```python
from build123d import *

# Parameters (mm, degrees)
SKETCH142_R               = 2.5
EXTRUDE046_DEPTH          = 19
EXTRUDE047_DEPTH          = 19
CYLINDER185_R             = 2
CYLINDER185_DEPTH         = 10
CYLINDER186_R             = 2
CYLINDER186_DEPTH         = 10
CYLINDER187_R             = 2
CYLINDER187_DEPTH         = 10
CYLINDER184_R             = 2
CYLINDER184_DEPTH         = 10
FUSION121_PLACEMENT_ANGLE = 45
CYLINDER180_R             = 2
CYLINDER180_DEPTH         = 10
CYLINDER181_R             = 2
CYLINDER181_DEPTH         = 10
CYLINDER182_R             = 2
CYLINDER182_DEPTH         = 10
CYLINDER183_R             = 2
CYLINDER183_DEPTH         = 10
CYLINDER170_R             = 2
CYLINDER170_DEPTH         = 10
CYLINDER171_R             = 2
CYLINDER171_DEPTH         = 10
CYLINDER172_R             = 2
CYLINDER172_DEPTH         = 10
CYLINDER169_R             = 2
CYLINDER169_DEPTH         = 10
FUSION111_PLACEMENT_ANGLE = 45
CYLINDER176_R             = 5
CYLINDER176_DEPTH         = 5.82
CYLINDER177_R             = 5
CYLINDER177_DEPTH         = 5.82
CYLINDER178_R             = 5
CYLINDER178_DEPTH         = 5.82
CYLINDER179_R             = 5
CYLINDER179_DEPTH         = 5.82
CYLINDER173_R             = 40
CYLINDER173_DEPTH         = 4.5
CYLINDER174_R             = 24
CYLINDER174_DEPTH         = 7
EXTRUDE044_DEPTH          = 33
SKETCH141_W               = 27
SKETCH141_H               = 14.5
SKETCH141_R               = 2.125
EXTRUDE045_DEPTH          = 4


with BuildPart() as lightwire:
    # Sketch142 → Extrude046 (new body)
    with BuildSketch(Plane.XY.offset(-24.25)):
        with Locations((18.5, -375)):
            Circle(SKETCH142_R)
    extrude(amount=EXTRUDE046_DEPTH)


with BuildPart() as extrude047:
    # Sketch143 → Extrude047 (new body)
    with BuildSketch(Plane.XY.offset(-24.25)):
        with BuildLine():
            ThreePointArc((18.5, -380), (23.5, -375), (18.5, -370))
            Line((13.5, -370), (18.5, -370))
            Line((13.5, -380), (13.5, -370))
            Line((18.5, -380), (13.5, -380))
        make_face()
    extrude(amount=EXTRUDE047_DEPTH)


with BuildPart() as obj1:
    # Cylinder185 → Cylinder185 (new body)
    with BuildSketch(Plane(origin=(35, 0, 65), x_dir=(1, 0, 0), z_dir=(0, 0, 1))):
        Circle(CYLINDER185_R)
    extrude(amount=CYLINDER185_DEPTH)


with BuildPart() as obj2:
    # Cylinder186 → Cylinder186 (new body)
    with BuildSketch(Plane(origin=(0, 35, 65), x_dir=(1, 0, 0), z_dir=(0, 0, 1))):
        Circle(CYLINDER186_R)
    extrude(amount=CYLINDER186_DEPTH)


with BuildPart() as obj3:
    # Cylinder187 → Cylinder187 (new body)
    with BuildSketch(Plane(origin=(0, -35, 65), x_dir=(1, 0, 0), z_dir=(0, 0, 1))):
        Circle(CYLINDER187_R)
    extrude(amount=CYLINDER187_DEPTH)


with BuildPart() as fusion121:
    # Cylinder184 → Cylinder184 (new body)
    with BuildSketch(Plane(origin=(-35, 0, 65), x_dir=(1, 0, 0), z_dir=(0, 0, 1))):
        Circle(CYLINDER184_R)
    extrude(amount=CYLINDER184_DEPTH)

    # Fusion121: union obj1, obj2, obj3
    add(obj1.part)
    add(obj2.part)
    add(obj3.part)


with BuildPart() as fusion121_1:
    # Fusion121 placement: moved
    add(fusion121.part.moved(Location((0, -374, -75))).rotate(Axis((0, -374, -75), (0, 0, -1)), FUSION121_PLACEMENT_ANGLE))


with BuildPart() as cylinder180:
    # Cylinder180 → Cylinder180 (new body)
    with BuildSketch(Plane(origin=(0, -21, 0), x_dir=(1, 0, 0), z_dir=(0, 0, 1))):
        Circle(CYLINDER180_R)
    extrude(amount=CYLINDER180_DEPTH)


with BuildPart() as m3heatsetcuts031:
    # Cylinder181 → Cylinder181 (new body)
    with BuildSketch(Plane(origin=(20.5, -21, 0), x_dir=(1, 0, 0), z_dir=(0, 0, 1))):
        Circle(CYLINDER181_R)
    extrude(amount=CYLINDER181_DEPTH)

    # Fusion118: union Cylinder180
    add(cylinder180.part)


with BuildPart() as m3heatsetcuts031_1:
    # Fusion118 placement: moved
    add(m3heatsetcuts031.part.moved(Location((-5, 39, 70))))


with BuildPart() as cylinder182:
    # Cylinder182 → Cylinder182 (new body)
    with BuildSketch(Plane(origin=(0, -21, 0), x_dir=(1, 0, 0), z_dir=(0, 0, 1))):
        Circle(CYLINDER182_R)
    extrude(amount=CYLINDER182_DEPTH)


with BuildPart() as m3heatsetcuts030:
    # Cylinder183 → Cylinder183 (new body)
    with BuildSketch(Plane(origin=(20.5, -21, 0), x_dir=(1, 0, 0), z_dir=(0, 0, 1))):
        Circle(CYLINDER183_R)
    extrude(amount=CYLINDER183_DEPTH)

    # Fusion119: union Cylinder182
    add(cylinder182.part)


with BuildPart() as m3heatsetcuts030_1:
    # Fusion119 placement: moved
    add(m3heatsetcuts030.part.moved(Location((-5, 3, 70))))

    # Fusion117: union m3HeatSetCuts031
    add(m3heatsetcuts031_1.part)


with BuildPart() as m3heatsetcuts030_2:
    # Fusion117 placement: moved
    add(m3heatsetcuts030_1.part.moved(Location((128.75, 10, -1))))


with BuildPart() as obj4:
    # Cylinder170 → Cylinder170 (new body)
    with BuildSketch(Plane(origin=(35, 0, 65), x_dir=(1, 0, 0), z_dir=(0, 0, 1))):
        Circle(CYLINDER170_R)
    extrude(amount=CYLINDER170_DEPTH)


with BuildPart() as obj5:
    # Cylinder171 → Cylinder171 (new body)
    with BuildSketch(Plane(origin=(0, 35, 65), x_dir=(1, 0, 0), z_dir=(0, 0, 1))):
        Circle(CYLINDER171_R)
    extrude(amount=CYLINDER171_DEPTH)


with BuildPart() as obj6:
    # Cylinder172 → Cylinder172 (new body)
    with BuildSketch(Plane(origin=(0, -35, 65), x_dir=(1, 0, 0), z_dir=(0, 0, 1))):
        Circle(CYLINDER172_R)
    extrude(amount=CYLINDER172_DEPTH)


with BuildPart() as fusion120:
    # Cylinder169 → Cylinder169 (new body)
    with BuildSketch(Plane(origin=(-35, 0, 65), x_dir=(1, 0, 0), z_dir=(0, 0, 1))):
        Circle(CYLINDER169_R)
    extrude(amount=CYLINDER169_DEPTH)

    # Fusion111: union obj4, obj5, obj6
    add(obj4.part)
    add(obj5.part)
    add(obj6.part)


with BuildPart() as fusion120_1:
    # Fusion111 placement: moved
    add(fusion120.part.moved(Location((0, -374, -75))).rotate(Axis((0, -374, -75), (0, 0, -1)), FUSION111_PLACEMENT_ANGLE))

    # Fusion120: union m3HeatSetCuts030
    add(m3heatsetcuts030_2.part)


with BuildPart() as cylinder176:
    # Cylinder176 → Cylinder176 (new body)
    with BuildSketch(Plane(origin=(0, -21, 0), x_dir=(1, 0, 0), z_dir=(0, 0, 1))):
        Circle(CYLINDER176_R)
    extrude(amount=CYLINDER176_DEPTH)


with BuildPart() as m3heatsetcuts027:
    # Cylinder177 → Cylinder177 (new body)
    with BuildSketch(Plane(origin=(20.5, -21, 0), x_dir=(1, 0, 0), z_dir=(0, 0, 1))):
        Circle(CYLINDER177_R)
    extrude(amount=CYLINDER177_DEPTH)

    # Fusion112: union Cylinder176
    add(cylinder176.part)


with BuildPart() as m3heatsetcuts027_1:
    # Fusion112 placement: moved
    add(m3heatsetcuts027.part.moved(Location((-5, 39, 70))))


with BuildPart() as cylinder178:
    # Cylinder178 → Cylinder178 (new body)
    with BuildSketch(Plane(origin=(0, -21, 0), x_dir=(1, 0, 0), z_dir=(0, 0, 1))):
        Circle(CYLINDER178_R)
    extrude(amount=CYLINDER178_DEPTH)


with BuildPart() as m3heatsetcuts029:
    # Cylinder179 → Cylinder179 (new body)
    with BuildSketch(Plane(origin=(20.5, -21, 0), x_dir=(1, 0, 0), z_dir=(0, 0, 1))):
        Circle(CYLINDER179_R)
    extrude(amount=CYLINDER179_DEPTH)

    # Fusion113: union Cylinder178
    add(cylinder178.part)


with BuildPart() as m3heatsetcuts029_1:
    # Fusion113 placement: moved
    add(m3heatsetcuts029.part.moved(Location((-5, 3, 70))))

    # Fusion114: union m3HeatSetCuts027
    add(m3heatsetcuts027_1.part)


with BuildPart() as m3heatsetcuts029_2:
    # Fusion114 placement: moved
    add(m3heatsetcuts029_1.part.moved(Location((128.75, 10, -1))))


with BuildPart() as base015:
    # Cylinder173 → Cylinder173 (new body)
    with BuildSketch(Plane(origin=(136, 0, 65), x_dir=(1, 0, 0), z_dir=(0, 0, 1))):
        Circle(CYLINDER173_R)
    extrude(amount=CYLINDER173_DEPTH)


with BuildPart() as basecut004:
    # Cylinder174 → Cylinder174 (new body)
    with BuildSketch(Plane(origin=(5, 0, 74), x_dir=(1, 0, 0), z_dir=(0, 0, 1))):
        Circle(CYLINDER174_R)
    extrude(amount=CYLINDER174_DEPTH)


with BuildPart() as lightmodule:
    # Sphere006 → Sphere006 (revolve)
    with BuildSketch(Plane(origin=(5, 0, 74), x_dir=(1, 0, 0), z_dir=(0, -1, 0))):
        with BuildLine():
            ThreePointArc((27.5, 0), (27.349352, 2.874533), (26.899059, 5.717571))
            Line((26.899059, 5.717571), (0, 5.717571))
            Line((0, 5.717571), (0, 0))
            Line((0, 0), (27.5, 0))
        make_face()
    revolve(axis=Axis((5, 0, 74), (0, 0, 1)))

    # Cut058: cut baseCut004
    add(basecut004.part, mode=Mode.SUBTRACT)


with BuildPart() as lightmodule_1:
    # Cut058 placement: moved
    add(lightmodule.part.moved(Location((131, 0, -5))))

    # Fusion115: union base015
    add(base015.part)


with BuildPart() as lightmodule_2:
    # Fusion115 placement: moved
    add(lightmodule_1.part.moved(Location((-2, 10, 0))))

    # Fusion116: union m3HeatSetCuts029
    add(m3heatsetcuts029_2.part)

    # Cut059: cut Fusion120
    add(fusion120_1.part, mode=Mode.SUBTRACT)


with BuildPart() as lightmodule_3:
    # Cut059 placement: moved
    add(lightmodule_2.part.moved(Location((-134, -384, -74.75))))

    # Cut060: cut Fusion121
    add(fusion121_1.part, mode=Mode.SUBTRACT)


with BuildPart() as extrude044:
    # Sketch140 → Extrude044 (new body)
    with BuildSketch(Plane.XZ.offset(370)):
        Polygon((-13.5, -9.75), (-9.5, -9.75), (-9.5, -20.25), (9.5, -20.25), (9.5, -9.75), (13.5, -9.75), (13.5, -24.25), (-13.5, -24.25), align=None)
    extrude(amount=EXTRUDE044_DEPTH)


with BuildPart() as lightmodule015:
    # Sketch141 → Extrude045 (new body)
    with BuildSketch(Plane.XZ.offset(403)):
        with Locations((0, -17)):
            Rectangle(SKETCH141_W, SKETCH141_H)
        with Locations((0, -15)):
            Circle(SKETCH141_R, mode=Mode.SUBTRACT)
    extrude(amount=EXTRUDE045_DEPTH)

    # Fusion122: union lightModule, Extrude044
    add(lightmodule_3.part)
    add(extrude044.part)

    # Fusion123: union Extrude047
    add(extrude047.part)

    # Cut061: cut lightWire
    add(lightwire.part, mode=Mode.SUBTRACT)


solid = lightmodule015.part
```
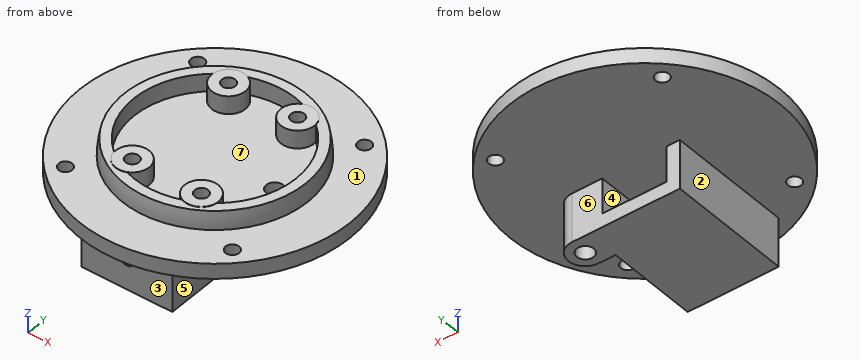
The model under review builds one solid part; all positions refer to its coordinate system, in mm. Face numbers are marked on the shaded views. A direction names the side the tool comes from. Give positions to 0.01 mm unless a question says otherwise; leave off trailing zeros. Write each loop counter-clockwise with the first axis right and the second up, starting at its lowest first coordinate (ties: lowest second). Pieces come first, ordered by that corner, then holes. Notation, with made-up numbers: (65, -13.5) -> (117, -13.5) arc R11 ccw to (117, 1.5) -> close; hole circle Ø5 at (74, 29). An arc over 180 degrees is marked (long way). Put each result on its own line as item: value.
(1) For pin 1 Ø4.5 at (x, y) = (-24.75, -349.25) entering from -Z; pin 2 Ø3 at (x, z) = (4, -4.5) entering from +Y; pin 3 Ø2 at (x, y) = (-28, -387.5) entering from +Z, all flat-tipped, find the tip position at first contact; note any pin that passes through.
Results are:
pin 1: z = -9.75
pin 2: y = -334.09
pin 3: z = -5.25
(2) We need section C-C, the plane y = -342. Give the boundary of the cut face in (x, z), and give its area (3 significant figures).
Results are:
outline: (-24, -9.75) -> (24, -9.75) -> (24, -5.25) -> (-24, -5.25) -> close
area: 216 mm²
(3) We need section B-B, the plane y = -375. State how many separate pieces and enclosed holes the cut face has, and give its area (3 significant figures).
Results are:
separate pieces: 2
enclosed holes: 1
area: 636 mm²
(4) The part is to be moulded in two halves that separate along X. For the marked faces 5, 6 and 7, say which applies: pulls with the +X half, pulls with the -X half, needs draft (parallel to the pull), parting line crosses it, or undercut.
Results are:
face 5: pulls with the +X half
face 6: needs draft
face 7: undercut
(5) We need section D-D, the plane x = 29.5. Give the boundary of the cut face in (y, z).
Results are:
outline: (-401.01, -9.75) -> (-346.99, -9.75) -> (-346.99, -5.25) -> (-401.01, -5.25) -> close
(6) To check wall thickness, follow probe 1 along Z at (x, y) = (-6, -388); probe 2 along Y at (x, z) = (-23.5, -7); probe 3 along Y at (x, z) = (18.5, -16). State the ranges of each line that lie inside material, in increasing order. Write a range as from..to.
Results are:
probe 1: -24.25..-20.25, -9.75..-5.25
probe 2: -406.37..-400.31, -397.19..-350.81, -347.69..-341.63
probe 3: -380..-377.5, -372.5..-370
(7) Tool access review of the marked faces 1, 2, 3 and 4: name each direction out of +Z, -Z, +X, -X, +Y, -Y from which nothing blocks a thin tool from reaching the whole face with its end or side.
Results are:
face 1: +Z
face 2: -Z, -X, +Y, -Y
face 3: -Z, +X, -X, -Y
face 4: +Y
(8) We need section A-A, the plane z = -7. Give the boundary of the cut face in (x, y), and give its area (3 significant figures).
Results are:
outline: circle Ø80 at (0, -374); hole circle Ø4 at (-24.75, -398.75); hole circle Ø4 at (-24.75, -349.25); hole circle Ø5 at (18.5, -375); hole circle Ø4 at (24.75, -398.75); hole circle Ø4 at (24.75, -349.25)
area: 4,960 mm²
